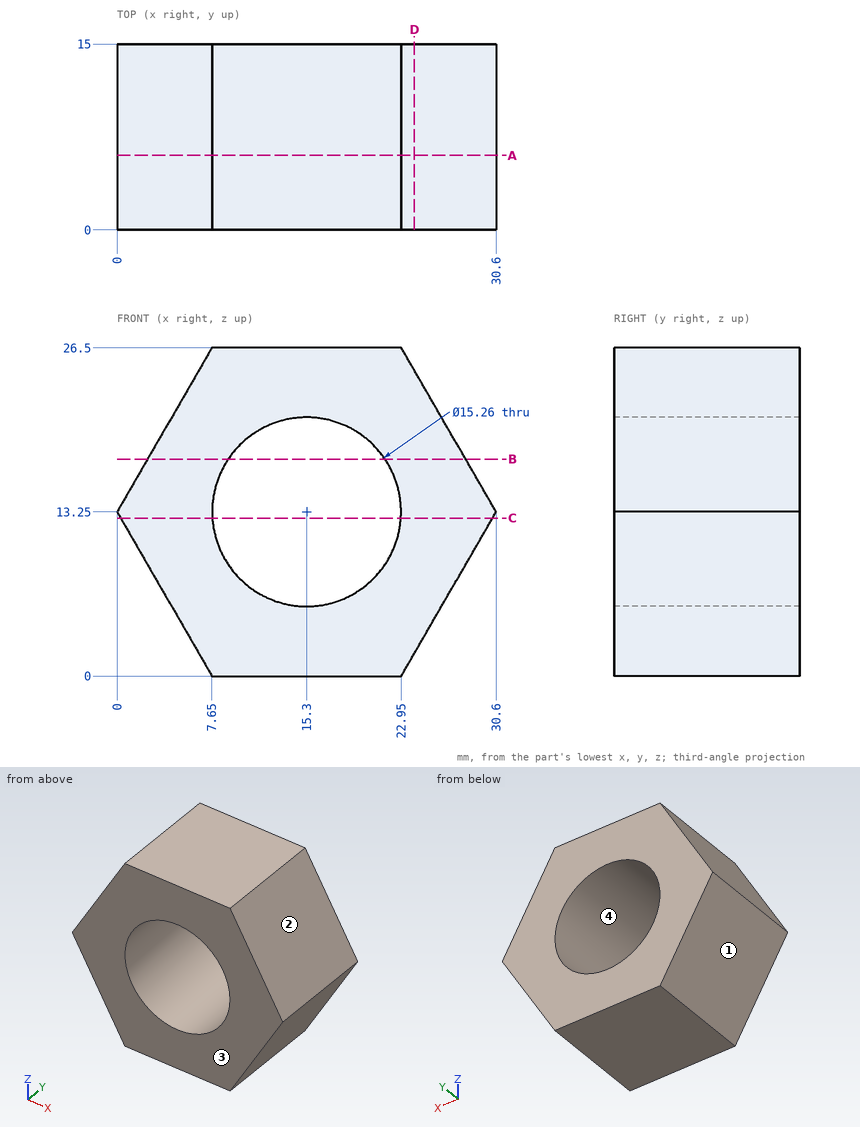
Geometry: see drawing. Coordinates: mm, zero at the bounding-box minimum. Round coordinates to 2 decimals unless told otherwise and drop trailing zeros. Write each loop counter-clockwise with the first axis right and the second up, starting at its lowest first coordinate (ties: lowest second). Pieces come first, ordered by that corner, then holes.
1) Cut plane B-B (z = 17.5). Return the cut outline in (x, y) (1 decimal).
2) Draft query along Z for the marked faces 1, 2, 3 and 4. Return one class per face: pulls with the +Z half, pulls with the -Z half, needs draft (parallel to the pull), parting line crosses it, or undercut.
3) Cut plane A-A (y = 6). Return the cut outline in (x, z).
4) Ray query, L1, parallel to Z at x = 15, y = 1.5 (1 decimal); L2, parallel to Z at x = 9, y = 5.75 (1 decimal); L3, parallel to X at y = 13.75, z = 14 (1 decimal). Return the intervals inside material, ascending.
5) Contact query for flat-ended pins moving along their axis: P1, Ø5, axis at y = 6.5, z = 10, coming from the -X side; P2, Ø5, axis at y = 1.5, z = 18.5, coming from the -X side; P3, Ø10, axis at x = 20.5, z = 5, coming from the -Y side; P4, Ø3, axis at x = 4.5, y = 9.5, coming from the +Z side (1 decimal). Output: stop coordinate, or through.
6) Cut plane D-D (x = 24). Return the cut outline in (y, z), then the cut area to 3 significant figures.
7) Cut plane C-C (z = 12.75). Return the cut outline in (x, y).
Geometry says:
1. outline: (2.5, 0) - (9, 0) - (9, 15) - (2.5, 15) - close; (21.6, 0) - (28.1, 0) - (28.1, 15) - (21.6, 15) - close
2. face 1: pulls with the -Z half
2. face 2: pulls with the +Z half
2. face 3: needs draft
2. face 4: undercut
3. outline: (0, 13.25) - (7.65, 0) - (22.95, 0) - (30.6, 13.25) - (22.95, 26.5) - (7.65, 26.5) - close; hole circle Ø15.26 at (15.3, 13.25)
4. L1: z = 0 to 5.6, 20.9 to 26.5
4. L2: z = 0 to 8.9, 17.6 to 26.5
4. L3: x = 0.4 to 7.7, 22.9 to 30.2
5. P1: stops at x = 0.43
5. P2: stops at x = 1.59
5. P3: stops at y = 0
5. P4: stops at z = 23.6
6. outline: (0, 1.82) - (15, 1.82) - (15, 24.68) - (0, 24.68) - close
6. area: 343 mm2
7. outline: (0.29, 0) - (7.69, 0) - (7.69, 15) - (0.29, 15) - close; (22.91, 0) - (30.31, 0) - (30.31, 15) - (22.91, 15) - close
